Check sheet for the modelled part. Datum: model origin and axes. Units: mm. A direction names the side the tool comes from. Coordinates: 2 decimals unless noted, no trailing zeros. Loops run counter-clockwise (first coordinate to the right, second up) from the corner with the lowest first, then second, coordinate; pieces in that order, holes last. Notation, with made-up numbers: (-20.5, -7.75) -> (20.5, -7.75) arc R16 ccw to (20.5, 17.25) -> close; hole circle Ø6 at (-31, 39.25). An arc over 180 degrees is marked (long way). Use CSV: the item, a comma, the result in double quotes.
```python
from build123d import *

# Parameters (mm, degrees)
BOSS_EXTRUDE1_DEPTH = 25.4
FILLET1_R           = 6.35
FILLET2_R           = 2.54


with BuildPart() as part:
    # Sketch1 → Boss-Extrude1 (new body)
    with BuildSketch(Plane.XY):
        Polygon((78.7654, -64.135), (88.9254, -64.135), (88.9254, 64.135), (-88.9254, 64.135), (-88.9254, -64.135), (-77.2414, -64.135), (-77.2414, 56.515), (78.7654, 56.515), align=None)
    extrude(amount=BOSS_EXTRUDE1_DEPTH)

    # Fillet1
    fillet1_edges = [part.edges().sort_by_distance(p)[0] for p in [
        (78.7654, 56.515, 12.7),
        (-77.2414, 56.515, 12.7),
    ]]
    fillet(fillet1_edges, radius=FILLET1_R)

    # Fillet2
    fillet2_edges = [part.edges().sort_by_distance(p)[0] for p in [
        (-88.9254, 64.135, 12.7),
        (88.9254, 64.135, 12.7),
    ]]
    fillet(fillet2_edges, radius=FILLET2_R)


solid = part.part
```
1) Access from +Z, -Z, +X, -X, +Y, -Y to the whole of each face (thin tool, end or side, straight path). Record for faces 4 (the cylindrical face through (-75.431, 54.605, 12.878)), 5 (the flat face through (1, 64.135, 13)).
Answer below:
face 4,"+Z, -Z, -Y"
face 5,"+Z, -Z, +X, -X, +Y"
2) Cross-section at D-D on x = 76. Record the boundary of the cut face in (y, z) (3 decimals).
Answer below:
outline,"(55.406, 0) -> (64.135, 0) -> (64.135, 25.4) -> (55.406, 25.4) -> close"
3) Go/stop test with a flat-tipped pin: pin 1 Ø7.5 at (x, z) = (-32.5, 8) entering from -Y (3 decimals). Record where the tip stops, or that it passes through.
Answer below:
pin 1,"stops at y = 56.515"
4) Cross-section at B-B on z = 3.25. Record the boundary of the cut face in (x, y) (3 decimals).
Answer below:
outline,"(-88.925, -64.135) -> (-77.241, -64.135) -> (-77.241, 50.165) arc R6.35 cw to (-70.891, 56.515) -> (72.415, 56.515) arc R6.35 cw to (78.765, 50.165) -> (78.765, -64.135) -> (88.925, -64.135) -> (88.925, 61.595) arc R2.54 ccw to (86.385, 64.135) -> (-86.385, 64.135) arc R2.54 ccw to (-88.925, 61.595) -> close"
5) Cross-section at C-C on x = 27.5. Record the boundary of the cut face in (y, z) (3 decimals).
Answer below:
outline,"(56.515, 0) -> (64.135, 0) -> (64.135, 25.4) -> (56.515, 25.4) -> close"
6) Cross-section at A-A on y = -46.5. Record the boundary of the cut face in (x, z).
Answer below:
outline,"(-88.93, 0) -> (-77.24, 0) -> (-77.24, 25.4) -> (-88.93, 25.4) -> close; (78.77, 0) -> (88.93, 0) -> (88.93, 25.4) -> (78.77, 25.4) -> close"
7) Thickness scan on line 1 along X through (y, z) = (-46.5, 10); line 2 along Y through (x, z) = (-31.5, 6) (3 decimals). Record the ranges inside material, lowest first. Write a range as from..to.
Answer below:
line 1,"x = -88.93..-77.24, 78.77..88.93"
line 2,"y = 56.515..64.135"
8) Draft check along X on faces 1 (the flat face through (-77.241, -8, 13)), 2 (the flat face through (-88.925, 0, 13)), 3 (the flat face through (-14, 57, 25.4)). Enter one of: released by +X, released by -X, zero draft, split by the parting line, or undercut.
Answer below:
face 1,"undercut"
face 2,"released by -X"
face 3,"zero draft"
